Source: CAD feature listing. Evaluate the final solid. Frame: model axes, mm. A direction names the side the tool comes from. Give positions to 0.01 mm unless a question says otherwise; leave off trailing zeros. Order: outer loops, then holes, each group sorted by start corner. A loop starts at its lowest first (then second) coordinate and runs counter-clockwise, first axis right, second up. Notation, with made-up numbers: (-39.75, 10) - (-26.75, 10) arc R21 ccw to (-26.75, 37) - close; hole circle Ø1 at (87, -27.5). An arc over 180 degrees is marked (long way). One line per item, written item: value. Start each with the question number.
from build123d import *

# Parameters (mm, degrees)
SKETCH1_R           = 20
SKETCH1_R_2         = 15
BOSS_EXTRUDE2_DEPTH = 10
SKETCH2_R           = 17
BOSS_EXTRUDE4_DEPTH = 5
SKETCH5_R           = 3
CUT_EXTRUDE2_DEPTH  = 33.015621187


with BuildPart() as part:
    # Sketch1 → Boss-Extrude2 (new body)
    # profile 1 of 10: a face of its own
    with BuildSketch(Plane.XY):
        Circle(SKETCH1_R)
        Circle(SKETCH1_R_2, mode=Mode.SUBTRACT)
    # profile 2 of 10: a face of its own
    with BuildSketch(Plane.XY):
        with BuildLine():
            ThreePointArc((-4.708142303, 13.714350005), (-2.386621559, 14.302238899), (0, 14.5))
            Line((0, 14.5), (0, 15))
            ThreePointArc((0, 15), (-2.468918854, 14.795419551), (-4.870492038, 14.187258626))
            Line((-4.870492038, 14.187258626), (-4.708142303, 13.714350005))
        make_face()
    # profile 3 of 10: a face of its own
    with BuildSketch(Plane.XY):
        with BuildLine():
            Line((9.21319069, 11.837107641), (8.906084334, 11.442537386))
            ThreePointArc((8.906084334, 11.442537386), (10.667996705, 9.820582789), (12.138913935, 7.930748293))
            Line((12.138913935, 7.930748293), (12.557497174, 8.204222372))
            ThreePointArc((12.557497174, 8.204222372), (11.03585866, 10.159223574), (9.21319069, 11.837107641))
        make_face()
    # profile 4 of 10: a face of its own
    with BuildSketch(Plane.XY):
        with BuildLine():
            Line((14.541003989, 3.682282307), (14.056303856, 3.559539564))
            ThreePointArc((14.056303856, 3.559539564), (14.388648406, 1.793543153), (14.5, 0))
            ThreePointArc((14.5, 0), (14.487613497, -0.599212127), (14.450475149, -1.197400509))
            Line((14.450475149, -1.197400509), (14.948767395, -1.238690182))
            ThreePointArc((14.948767395, -1.238690182), (14.987186376, -0.619874614), (15, 0))
            ThreePointArc((15, 0), (14.884808696, 1.855389469), (14.541003989, 3.682282307))
        make_face()
    # profile 5 of 10: a face of its own
    with BuildSketch(Plane.XY):
        with BuildLine():
            Line((13.7365999, -6.02543137), (13.278713236, -5.824583657))
            ThreePointArc((13.278713236, -5.824583657), (12.138913935, -7.930748293), (10.667996705, -9.820582789))
            Line((10.667996705, -9.820582789), (11.03585866, -10.159223574))
            ThreePointArc((11.03585866, -10.159223574), (12.557497174, -8.204222372), (13.7365999, -6.02543137))
        make_face()
    # profile 6 of 10: a face of its own
    with BuildSketch(Plane.XY):
        with BuildLine():
            Line((7.139210896, -13.192106268), (6.901237199, -12.752369392))
            ThreePointArc((6.901237199, -12.752369392), (4.708142303, -13.714350005), (2.386621559, -14.302238899))
            Line((2.386621559, -14.302238899), (2.468918854, -14.795419551))
            ThreePointArc((2.468918854, -14.795419551), (4.870492038, -14.187258626), (7.139210896, -13.192106268))
        make_face()
    # profile 7 of 10: a face of its own
    with BuildSketch(Plane.XY):
        with BuildLine():
            Line((-2.468918854, -14.795419551), (-2.386621559, -14.302238899))
            ThreePointArc((-2.386621559, -14.302238899), (-4.708142303, -13.714350005), (-6.901237199, -12.752369392))
            Line((-6.901237199, -12.752369392), (-7.139210896, -13.192106268))
            ThreePointArc((-7.139210896, -13.192106268), (-4.870492038, -14.187258626), (-2.468918854, -14.795419551))
        make_face()
    # profile 8 of 10: a face of its own
    with BuildSketch(Plane.XY):
        with BuildLine():
            Line((-11.03585866, -10.159223574), (-10.667996705, -9.820582789))
            ThreePointArc((-10.667996705, -9.820582789), (-12.138913935, -7.930748293), (-13.278713236, -5.824583657))
            Line((-13.278713236, -5.824583657), (-13.7365999, -6.02543137))
            ThreePointArc((-13.7365999, -6.02543137), (-12.557497174, -8.204222372), (-11.03585866, -10.159223574))
        make_face()
    # profile 9 of 10: a face of its own
    with BuildSketch(Plane.XY):
        with BuildLine():
            Line((-14.948767395, -1.238690182), (-14.450475149, -1.197400509))
            ThreePointArc((-14.450475149, -1.197400509), (-14.450475149, 1.197400509), (-14.056303856, 3.559539564))
            Line((-14.056303856, 3.559539564), (-14.541003989, 3.682282307))
            ThreePointArc((-14.541003989, 3.682282307), (-14.948767395, 1.238690182), (-14.948767395, -1.238690182))
        make_face()
    # profile 10 of 10: a face of its own
    with BuildSketch(Plane.XY):
        with BuildLine():
            Line((-12.557497174, 8.204222372), (-12.138913935, 7.930748293))
            ThreePointArc((-12.138913935, 7.930748293), (-10.667996705, 9.820582789), (-8.906084334, 11.442537386))
            Line((-8.906084334, 11.442537386), (-9.21319069, 11.837107641))
            ThreePointArc((-9.21319069, 11.837107641), (-11.03585866, 10.159223574), (-12.557497174, 8.204222372))
        make_face()
    extrude(amount=BOSS_EXTRUDE2_DEPTH)

    # Sketch2 → Boss-Extrude4 (add)
    with BuildSketch(Plane.XY):
        Circle(SKETCH2_R)
    extrude(amount=-BOSS_EXTRUDE4_DEPTH)

    # Sketch5 → Cut-Extrude2 (cut, through all)
    with BuildSketch(Plane(origin=(0, 0, -5), x_dir=(-1, 0, 0), z_dir=(0, 0, -1))):
        Circle(SKETCH5_R)
    extrude(amount=-CUT_EXTRUDE2_DEPTH, mode=Mode.SUBTRACT)


solid = part.part
1. Section D-D on x = -16. Return the cut outline in (y, z), then the cut area to 3 significant figures.
2. Section A-A on x = -0.5. Return the cut outline in (y, z).
3. Contact query for flat-ended pins moving along their axis: pin 1 Ø3 at (x, y) = (-3, 6.5) entering from +Z; pin 2 Ø5 at (x, y) = (14.5, -11.5) entering from -Z; pin 3 Ø3 at (y, z) = (15.5, 7) entering from +X; pin 4 Ø4 at (x, z) = (-7, 3) entering from -Y. Output: stop coordinate, or through.
4. Draft query along X for faces 1 (the flat face through (-12, -9, 10)), 2 (the cylindrical face through (9.139, 14.334, -2.465)), 3 (the cylindrical face through (-13.72, 6.06, 4.93)), 4 (the cylindrical face through (-10.691, 9.796, 4.93)). Return one class per face: pulls with the +X half, pulls with the -X half, needs draft (parallel to the pull), parting line crosses it, or undercut.
5. Set-up query: faces 5 (the cylindrical face through (3, 0, -3)), 6 (the flat face through (0, 4, 0)), 7 (the flat face through (-9, -15, 0)). Return all of +Z, -Z, +X, -X, +Y, -Y with unobstructed straight access to the full face (end or side cutting, diameter ignored); none if empty.
6. Section C-C on z = -3.25. Return the cut outline in (x, y), then the cut area to 3 significant figures.
7. Section B-B on y = -2.5. Return the cut outline in (x, z).
8. Ray query, L1, parallel to Y at x = 0, z = -1.15; L2, parallel to Y at x = -1, z = 9.25; L3, parallel to X at y = -5, z = 0.5. Return the intervals inside material, ascending.
Data:
1. outline: (-12, 0) - (-5.74, 0) - (-5.74, -5) - (5.74, -5) - (5.74, 0) - (12, 0) - (12, 10) - (-12, 10) - close
1. area: 297 mm2
2. outline: (-19.99, 0) - (-16.99, 0) - (-16.99, -5) - (-2.96, -5) - (-2.96, 0) - (-14.99, 0) - (-14.99, 10) - (-19.99, 10) - close; (2.96, -5) - (16.99, -5) - (16.99, 0) - (19.99, 0) - (19.99, 10) - (14.49, 10) - (14.49, 0) - (2.96, 0) - close
3. pin 1: stops at z = 0
3. pin 2: stops at z = -5
3. pin 3: stops at x = 14.28
3. pin 4: stops at y = -19.36
4. face 1: needs draft
4. face 2: parting line crosses it
4. face 3: undercut
4. face 4: undercut
5. face 5: +Z, -Z
5. face 6: +Z
5. face 7: -Z
6. outline: circle Ø34 at (0, 0); hole circle Ø6 at (0, 0)
6. area: 880 mm2
7. outline: (-19.84, 0) - (-16.82, 0) - (-16.82, -5) - (-1.66, -5) - (-1.66, 0) - (-14.79, 0) - (-14.79, 10) - (-19.84, 10) - close; (1.66, -5) - (16.82, -5) - (16.82, 0) - (19.84, 0) - (19.84, 10) - (14.79, 10) - (14.79, 0) - (1.66, 0) - close
8. L1: y = -17 to -3, 3 to 17
8. L2: y = -19.97 to -14.97, 14.47 to 19.97
8. L3: x = -19.36 to -14.14, 14.14 to 19.36
